The model under review builds one solid part; all positions refer to its coordinate system, in mm. Coordinates: 2 decimals unless noted, no trailing zeros. Write each loop counter-clockwise with the first axis right and the second up, starting at its lowest first coordinate (ties: lowest second). Pieces come first, ordered by that corner, then holes. Notation, with made-up numbers: (88, 73) - (107, 73) arc R29 ccw to (107, 105) - close; hole circle Ø4 at (5, 49). An arc over 180 degrees is marked (long way). Answer as CSV lines item,"result". Start each with the question number.
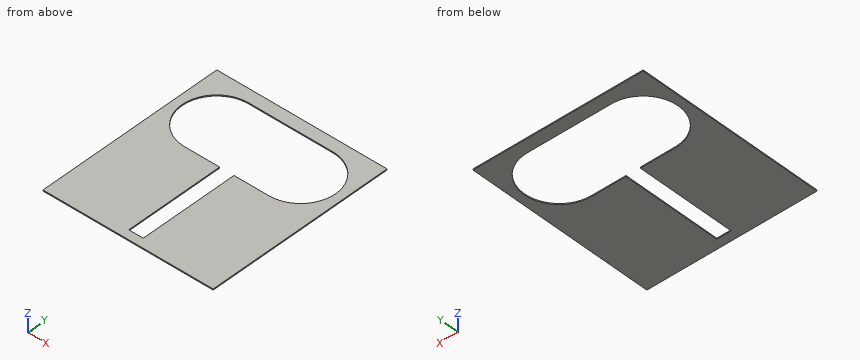
```python
from build123d import *

# Parameters (mm, degrees)
F1_DEPTH = 1


with BuildPart() as f1:
    # F0 (on Top) → F1 (new body)
    with BuildSketch(Plane.XY):
        Polygon((79.570077, 44.001997), (0, 44.001997), (-79.570077, 44.001997), (-79.570077, -133.093104), (0, -133.093104), (79.570077, -133.093104), align=None)
        with BuildLine():
            Line((-37.90909, 32.472326), (39.238343, 32.499998))
            ThreePointArc((39.238343, 32.499998), (62.226849, 22.985092), (71.75, 0))
            ThreePointArc((71.75, 0), (62.230607, -22.981334), (39.248972, -32.5))
            Line((39.248972, -32.5), (6.75, -32.498972))
            Line((6.75, -32.498972), (6.75, -125))
            Line((6.75, -125), (-6.75, -125))
            Line((-6.75, -125), (-6.75, -32.498545))
            Line((-6.75, -32.498545), (-38.849285, -32.49753))
            ThreePointArc((-38.849285, -32.49753), (-39.251028, -32.5), (-39.652771, -32.497504))
            ThreePointArc((-39.652771, -32.497504), (-71.746442, -0.480895), (-40.614204, 32.471356))
            ThreePointArc((-40.614204, 32.471356), (-39.261657, 32.499998), (-37.90909, 32.472326))
        make_face(mode=Mode.SUBTRACT)
    extrude(amount=F1_DEPTH)


solid = f1.part
```
(1) Add section A-A on y = -88.5. Give the boundary of the cut face in (x, z).
(2) Add section B-B on z = 0.4. Give the boundary of the cut face in (x, y), then the cut area to 3 significant figures.
(3) Add section C-C on x = 20.5. Give the boundary of the cut face in (y, z).
(4) Wall thickness on line 1 (X direction, y = -105.5, z = 0.75); line 2 (Y direction, x = -37, z = 0.8); line 3 (Y direction, x = -1.5, z = 0.85): over which ranges is each line inside the solid? List them lowest first.
Reported:
1,outline,"(-79.57, 0) - (-6.75, 0) - (-6.75, 1) - (-79.57, 1) - close; (6.75, 0) - (79.57, 0) - (79.57, 1) - (6.75, 1) - close"
2,outline,"(-79.57, -133.09) - (79.57, -133.09) - (79.57, 44) - (-79.57, 44) - close; hole (-40.61, 32.47) arc R32.5 ccw to (-39.65, -32.5) arc R32.5 ccw to (-38.85, -32.5) - (-6.75, -32.5) - (-6.75, -125) - (6.75, -125) - (6.75, -32.5) - (39.25, -32.5) arc R32.5 ccw to (71.75, 0) arc R32.5 ccw to (39.24, 32.5) - (-37.91, 32.47) arc R32.5 ccw to start"
2,area,"18,500 mm²"
3,outline,"(-133.09, 0) - (-32.5, 0) - (-32.5, 1) - (-133.09, 1) - close; (32.49, 0) - (44, 0) - (44, 1) - (32.49, 1) - close"
4,line 1,"-79.57 to -6.75, 6.75 to 79.57"
4,line 2,"-133.09 to -32.5, 32.47 to 44"
4,line 3,"-133.09 to -125, 32.49 to 44"
